Input: dimensioned drawing with shaded views. Units: mm. Origin: part minimum x, y, z. Round coordinates to 2 decimals unless told otherwise and drop trailing zeros. Loops run counter-clockwise (first coordinate to the right, second up) from the corner with the lowest first, then second, coordinate; pieces in that order, holes last. Notation, with made-up numbers: (27.5, 2) - (74.5, 2) arc R18 ccw to (74.5, 19) - close; hole circle Ø4 at (-20.75, -14). An arc over 180 degrees is marked (long way). One line per question, with ' | ' between items. Start each with the question number.
1. Ray query, line 1 (Z direction, x = 15, y = 2.8) (1 decimal); line 2 (Z direction, x = 20, y = 1.8); line 3 (Z direction, x = 23.5, y = 1.3). Return the intervals inside material, ascending.
2. Pin query (flat end, axial travel): pin 1 (1.9 mm diameter, centred on x = 16, z = 26.93, fed in from +Y); pin 2 (1.5 mm diameter, centred on x = 11, y = 1.5, fed in from -Z); pin 3 (3.5 mm diameter, centred on x = 24, z = 26.93, fed in from +Y); pin 4 (1 mm diameter, centred on y = 1, z = 25, fed in from +X). Return the tip coordinate at first contact, or that it passes through.
3. Cut plane B-B (z = 20). Return loops of the section in (x, y).
4. Mould query, pull axis Z, two halves, no side actions, for the marked faces 1, 2 and 3. Classes: pulls with the +Z half, pulls with the -Z half, needs draft (parallel to the pull), parting line crosses it, or undercut.
5. Cut plane D-D (y = 1.5). State how many separate pieces and enclosed holes the cut face has, then the cut area to 3 significant figures.
6. Cut plane A-A (x = 20). Return loops of the section in (y, z).
7. Cut plane C-C (x = 16). Return loops of the section in (y, z).
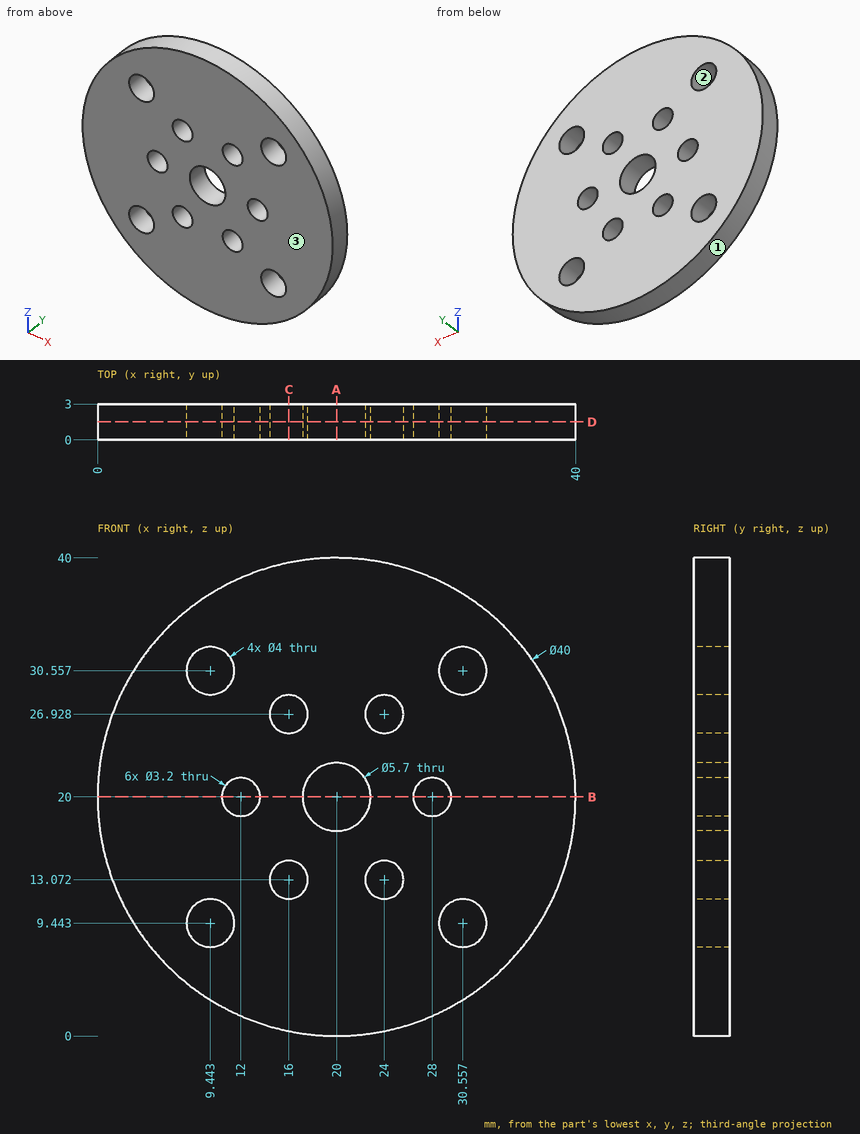
Answers follow:
1) line 1: z = 0.6 to 11.8, 14.3 to 25.7, 28.2 to 39.4 | line 2: z = 0 to 17.15, 22.85 to 40 | line 3: z = 0.31 to 11.55, 14.59 to 25.41, 28.45 to 39.69
2) pin 1: passes through | pin 2: stops at z = 1.78 | pin 3: stops at y = 3 | pin 4: stops at x = 39.49
3) outline: (0, 0) - (10.4, 0) - (10.4, 3) - (0, 3) - close; (13.6, 0) - (17.15, 0) - (17.15, 3) - (13.6, 3) - close; (22.85, 0) - (26.4, 0) - (26.4, 3) - (22.85, 3) - close; (29.6, 0) - (40, 0) - (40, 3) - (29.6, 3) - close
4) face 1: parting line crosses it | face 2: undercut | face 3: needs draft
5) separate pieces: 1 | enclosed holes: 11 | area: 1,130 mm2
6) outline: (0, 0) - (3, 0) - (3, 17.15) - (0, 17.15) - close; (0, 22.85) - (3, 22.85) - (3, 40) - (0, 40) - close
7) outline: (0, 0.4) - (3, 0.4) - (3, 11.47) - (0, 11.47) - close; (0, 14.67) - (3, 14.67) - (3, 25.33) - (0, 25.33) - close; (0, 28.53) - (3, 28.53) - (3, 39.6) - (0, 39.6) - close
